Part model, mm, in its own coordinate system. Face numbers are marked on the shaded views. A direction names the side the tool comes from. Give positions to 0.01 mm unless a question says otherwise; leave off trailing zeros. Order: outer loops, then holes, each group sorted by start corner. A loop starts at its lowest first (then second) coordinate and runs counter-clockwise, first axis right, second up. Notation, with made-up numbers: (31.25, 54) - (83.25, 54) arc R22 cw to (83.25, 64) - close; hole circle Ø11 at (-12.75, 14). An arc over 180 degrees is marked (long way). Use one line per item in the form item = value. Start each with the question number.
1. Drill centre lines: line 1 (Y direction, x = 95, z = 2.9); line 2 (X direction, y = 86.5, z = 19.75); line 3 (Y direction, x = 70, z = 1.9). Where is each one in solid material? Low to high.
2. Band-saw the part on A-A, the plane z = 13. List the corners of the cut face in (x, y), plus the area to 3 significant figures.
3. Pin check, flat tips, straight feed: P1, Ø12, axis at x = 84.5, y = 58.5, coming from the +Z side; P2, Ø0.9, axis at x = 133.5, z = 7.5, coming from the -Y side; P3, Ø3.5, axis at y = 90, z = 5.5, coming from the -X side. Stop position of each tip, or through.
4. Tool access for the marked faces 1 and 2: list every direction of +Z, -Z, +X, -X, +Y, -Y with a clear straight run to the whole face (end or side of a thin tool).
5. Band-saw the part on C-C, the plane x = 140. List the corners of the cut face in (y, z), plus the area to 3 significant figures.
6. Band-saw the part on B-B, the plane y = 30. List the corners of the cut face in (x, z).
7. Band-saw the part on D-D, the plane x = 55. List the corners of the cut face in (y, z).
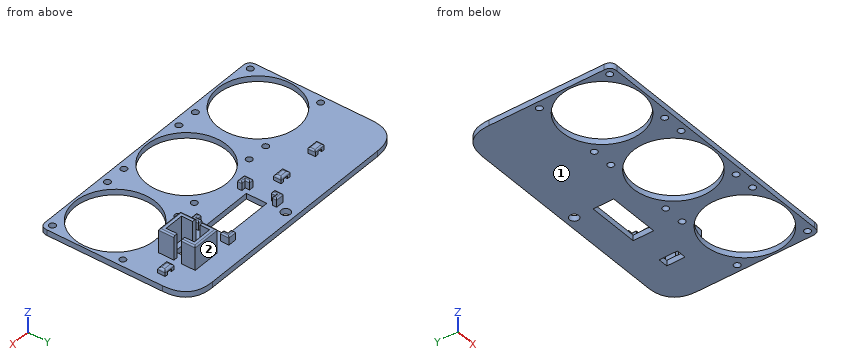
from build123d import *

# Parameters (mm, degrees)
F0_R         = 28.5
F1_DEPTH     = 4
F2_D         = 6.5
F3_D         = 4.5
F5_DEPTH     = 17
F6_DEPTH     = 6
F4_W         = 36.4
F4_H         = 14.6
F7_DEPTH     = 25
F4_W_2       = 7
F4_H_2       = 13
F8_DEPTH     = 25
F9_T1_DEPTH  = 104
F10_T1_DEPTH = 29
F4_W_3       = 8
F4_H_3       = 5.3025707603
F4_H_4       = 5.3
F11_DEPTH    = 4
F12_W        = 3.5351514816
F12_H        = 2
F13_DEPTH    = 25
F14_R        = 1.5
F15_R        = 1
F16_W        = 3.5
F16_H        = 2
F17_DEPTH    = 25
F18_R        = 1.5
F19_W        = 3.5
F19_H        = 2
F20_DEPTH    = 25
F21_R        = 1
F22_R        = 1


# Not quite as in the source:
# - a fillet or chamfer that OpenCascade refuses, or shapes differently, is made with other operations: its cross-section is extruded or revolved along the edge and cut away or added


with BuildPart() as f1:
    # F0 (on Top) → F1 (new body)
    with BuildSketch(Plane.XY):
        Polygon((0, 60), (0, 0), (60, 0), (65, 0), (125, 0), (130, 0), (190, 0), (190, 60), (190, 107), (0, 107), align=None)
        with Locations((30, 30)):
            Circle(F0_R, mode=Mode.SUBTRACT)
        with Locations((95, 30)):
            Circle(F0_R, mode=Mode.SUBTRACT)
        with Locations((160, 30)):
            Circle(F0_R, mode=Mode.SUBTRACT)
    extrude(amount=F1_DEPTH)

    # F2 (through all)
    with Locations(Plane(origin=(0, 0, 0), x_dir=(1, 0, 0), z_dir=(0, 0, -1))):
        with Locations((95, -100.5)):
            Hole(F2_D / 2)

    # F3 (through all)
    with Locations(Plane(origin=(0, 0, 0), x_dir=(1, 0, 0), z_dir=(0, 0, -1))):
        with Locations((5, -55), (55, -55), (5, -5), (55, -5), (70, -55), (70, -5), (120, -5), (120, -55), (135, -55), (135, -5), (185, -5), (185, -55)):
            Hole(F3_D / 2)

    # F4 (on face) → F5 (join)
    with BuildSketch(Plane.XY.offset(4)):
        Polygon((150.7997452021, 83.1751078367), (150.7997452021, 90), (164.7997452021, 90), (164.7997452021, 83.1751078367), (167.7997452021, 83.1751078367), (167.7997452021, 93), (147.7997452021, 93), (147.7997452021, 83.1751078367), align=None)
        Polygon((150.7997452021, 70), (150.7997452021, 77.8725370765), (147.7997452021, 77.8725370765), (147.7997452021, 67), (167.7997452021, 67), (167.7997452021, 77.8725370765), (164.7997452021, 77.8725370765), (164.7997452021, 70), align=None)
    extrude(amount=F5_DEPTH)

    # F4 (on face) → F6 (join)
    with BuildSketch(Plane.XY.offset(4)):
        Polygon((132.2073462009, 93.8), (132.2073462009, 90.8), (135.2073462009, 90.8), (135.2073462009, 87.8), (138.2073462009, 87.8), (138.2073462009, 93.8), align=None)
        Polygon((138.2073462009, 66.2), (138.2073462009, 72.2), (135.2073462009, 72.2), (135.2073462009, 69.2), (132.2073462009, 69.2), (132.2073462009, 66.2), align=None)
        Polygon((88.8073462009, 66.2), (94.8073462009, 66.2), (94.8073462009, 69.2), (91.8073462009, 69.2), (91.8073462009, 72.2), (88.8073462009, 72.2), align=None)
        Polygon((88.8073462009, 87.8), (91.8073462009, 87.8), (91.8073462009, 90.8), (94.8073462009, 90.8), (94.8073462009, 93.8), (88.8073462009, 93.8), align=None)
    extrude(amount=F6_DEPTH)

    # F4 (on face) → F7 (cut)
    with BuildSketch(Plane.XY.offset(4)):
        with Locations((113.5073462009, 80)):
            Rectangle(F4_W, F4_H)
    extrude(amount=-F7_DEPTH, mode=Mode.SUBTRACT)

    # F4 (on face) → F8 (cut)
    with BuildSketch(Plane.XY.offset(4)):
        with Locations((157.7997452021, 80)):
            Rectangle(F4_W_2, F4_H_2)
    extrude(amount=-F8_DEPTH, mode=Mode.SUBTRACT)

    # F9: fillet of radius 20 on 2 edges, made by hand

    # F9_s2 → F9_t1 (cut)
    with BuildSketch(Plane.XY.offset(-50)):
        with BuildLine():
            add(Edge.make_bspline(
                [(0, 87), (0, 107), (20, 107)],
                knots=[0, 0, 0, 1, 1, 1], degree=2, weights=[1, 1, 1]))
            Line((20, 107), (0, 107))
            Line((0, 107), (0, 87))
        make_face()
        with BuildLine():
            add(Edge.make_bspline(
                [(170, 107), (190, 107), (190, 87)],
                knots=[0, 0, 0, 1, 1, 1], degree=2, weights=[1, 1, 1]))
            Line((190, 87), (190, 107))
            Line((190, 107), (170, 107))
        make_face()
    extrude(amount=F9_T1_DEPTH, mode=Mode.SUBTRACT)

    # F10: fillet of radius 5 on 2 edges, made by hand

    # F10_s2 → F10_t1 (cut)
    with BuildSketch(Plane.XY.offset(-12.5)):
        with BuildLine():
            add(Edge.make_bspline(
                [(0, 5), (0, 0), (5, 0)],
                knots=[0, 0, 0, 1, 1, 1], degree=2, weights=[1, 1, 1]))
            Line((5, 0), (0, 0))
            Line((0, 0), (0, 5))
        make_face()
        with BuildLine():
            add(Edge.make_bspline(
                [(185, 0), (190, 0), (190, 5)],
                knots=[0, 0, 0, 1, 1, 1], degree=2, weights=[1, 1, 1]))
            Line((190, 5), (190, 0))
            Line((190, 0), (185, 0))
        make_face()
    extrude(amount=F10_T1_DEPTH, mode=Mode.SUBTRACT)

    # F4 (on face) → F11 (join)
    with BuildSketch(Plane.XY.offset(4)):
        with Locations((178.55278337, 80.5238224566)):
            Rectangle(F4_W_3, F4_H_3)
        with Locations((72.4365121722, 80.0548492312)):
            Rectangle(F4_W_3, F4_H_4)
        with Locations((41.3649373651, 80.0548492312)):
            Rectangle(F4_W_3, F4_H_4)
    extrude(amount=F11_DEPTH)

    # F12 (on face) → F13 (cut)
    with BuildSketch(Plane.XZ.offset(-77.8725370765)):
        with Locations((178.4631460905, 5)):
            Rectangle(F12_W, F12_H)
    extrude(amount=-F13_DEPTH, mode=Mode.SUBTRACT)

    # F14
    f14_edges = [f1.edges().sort_by_distance(p)[0] for p in [
        (174.552783, 80.523822, 8),
        (182.552783, 80.523822, 8),
        (178.552783, 83.175108, 8),
        (178.552783, 77.872537, 8),
    ]]
    fillet(f14_edges, radius=F14_R)

    # F15
    f15_edges = [f1.edges().sort_by_distance(p)[0] for p in [
        (147.799745, 72.436269, 21),
        (157.799745, 67, 21),
        (167.799745, 72.436269, 21),
        (147.799745, 88.087554, 21),
        (157.799745, 93, 21),
        (167.799745, 88.087554, 21),
    ]]
    fillet(f15_edges, radius=F15_R)

    # F16 (on face) → F17 (cut)
    with BuildSketch(Plane.XZ.offset(-77.4048492312)):
        with Locations((72.4831895828, 5)):
            Rectangle(F16_W, F16_H)
    extrude(amount=-F17_DEPTH, mode=Mode.SUBTRACT)

    # F18
    f18_edges = [f1.edges().sort_by_distance(p)[0] for p in [
        (72.436512, 82.704849, 8),
        (68.436512, 80.054849, 8),
        (72.436512, 77.404849, 8),
        (76.436512, 80.054849, 8),
    ]]
    fillet(f18_edges, radius=F18_R)

    # F19 (on face) → F20 (cut)
    with BuildSketch(Plane.XZ.offset(-77.4048492312)):
        with Locations((41.3242319524, 5)):
            Rectangle(F19_W, F19_H)
    extrude(amount=-F20_DEPTH, mode=Mode.SUBTRACT)

    # F21
    f21_edges = [f1.edges().sort_by_distance(p)[0] for p in [
        (41.364937, 77.404849, 8),
        (45.364937, 80.054849, 8),
        (41.364937, 82.704849, 8),
        (37.364937, 80.054849, 8),
    ]]
    fillet(f21_edges, radius=F21_R)

    # F22
    f22_edges = [f1.edges().sort_by_distance(p)[0] for p in [
        (90.307346, 87.8, 10),
        (91.807346, 89.3, 10),
        (93.307346, 90.8, 10),
        (94.807346, 92.3, 10),
        (91.807346, 93.8, 10),
        (88.807346, 90.8, 10),
        (132.207346, 92.3, 10),
        (133.707346, 90.8, 10),
        (135.207346, 89.3, 10),
        (136.707346, 87.8, 10),
        (138.207346, 90.8, 10),
        (135.207346, 93.8, 10),
        (138.207346, 69.2, 10),
        (136.707346, 72.2, 10),
        (135.207346, 70.7, 10),
        (133.707346, 69.2, 10),
        (132.207346, 67.7, 10),
        (135.207346, 66.2, 10),
        (91.807346, 66.2, 10),
        (94.807346, 67.7, 10),
        (93.307346, 69.2, 10),
        (91.807346, 70.7, 10),
        (90.307346, 72.2, 10),
        (88.807346, 69.2, 10),
    ]]
    fillet(f22_edges, radius=F22_R)


solid = f1.part
From the geometry:
q1.line_1 = 0 to 1.5, 58.5 to 97.25, 103.75 to 107
q1.line_2 = 147.8 to 150.8, 164.8 to 167.8
q1.line_3 = 0 to 2.75, 7.25 to 16.32, 43.68 to 52.75, 57.25 to 107
q2.outline = (147.8, 67) - (167.8, 67) - (167.8, 77.87) - (164.8, 77.87) - (164.8, 70) - (150.8, 70) - (150.8, 77.87) - (147.8, 77.87) - close; (147.8, 83.18) - (150.8, 83.18) - (150.8, 90) - (164.8, 90) - (164.8, 83.18) - (167.8, 83.18) - (167.8, 93) - (147.8, 93) - close
q2.area = 208 mm²
q3.P1 = 4
q3.P2 = 66.2
q3.P3 = 0.06
q4.face_1 = -Z, +X, -X, +Y, -Y
q4.face_2 = +Z, +X, +Y
q5.outline = (0, 0) - (9.7, 0) - (9.7, 4) - (0, 4) - close; (50.3, 0) - (107, 0) - (107, 4) - (50.3, 4) - close
q5.area = 266 mm²
q6.outline = (0, 0) - (1.5, 0) - (1.5, 4) - (0, 4) - close; (58.5, 0) - (66.5, 0) - (66.5, 4) - (58.5, 4) - close; (123.5, 0) - (131.5, 0) - (131.5, 4) - (123.5, 4) - close; (188.5, 0) - (190, 0) - (190, 4) - (188.5, 4) - close
q7.outline = (0, 0) - (2.75, 0) - (2.75, 4) - (0, 4) - close; (7.25, 0) - (16.32, 0) - (16.32, 4) - (7.25, 4) - close; (43.68, 0) - (52.75, 0) - (52.75, 4) - (43.68, 4) - close; (57.25, 0) - (107, 0) - (107, 4) - (57.25, 4) - close
